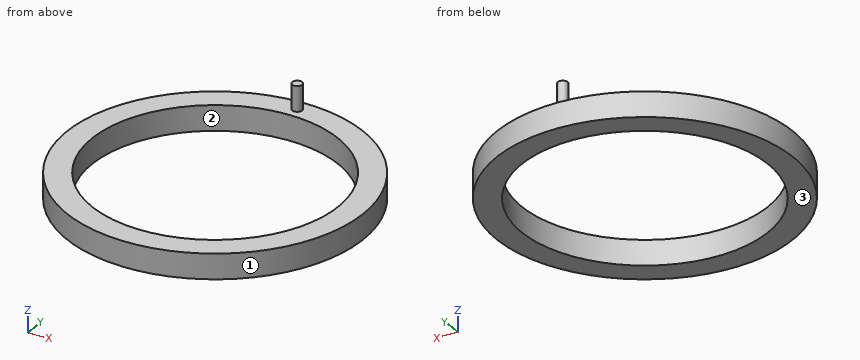
Autodesk Fusion 360 part; units mm, degrees
sketch "Sketch1" plane through (0, 0, 0) normal (0, 0, 1) x (1, 0, 0)
  circle A0 centre (0, 0) radius 29.5
  dimension "d1" = 59
sketch "Sketch2" plane through (0, 0, 0) normal (0, 0, 1) x (1, 0, 0)
  circle A0 centre (0, 0) radius 22.5
  dimension "d2" = 45
extrude "Extrude1" add sketch "Sketch1" sketch "Sketch2" along normal blind 5 of sketch 2
sketch "Sketch3" plane through (0, 0, 5) normal (0, 0, 1) x (-1, 0, 0)
  circle A0 centre (0, 0) radius 29.5
  circle A1 centre (0, 0) radius 24.5
  dimension "d5" = 49
extrude "Extrude2" cut sketch "Sketch3" against normal blind 115 contours A1
sketch "Sketch4" plane through (0, 0, 0) normal (0, 0, 1) x (1, 0, 0)
sketch "Sketch5" plane through (0, 0, 5) normal (0, 0, 1) x (-1, 0, 0)
  circle A0 centre (0, 0) radius 24.5
  circle A1 centre (0, 0) radius 29.5
  circle A2 centre (0, -27) radius 1
extrude "Extrude3" add sketch "Sketch5" along normal blind 5 contours A2
sketch "Sketch6" plane through (0, 0, 0) normal (0, 0, 1) x (1, 0, 0)
Here's how the part is built. I have some questions about the finished solid (model axes, mm). Face numbers are marked on the shaded views. Round coordinates to 2 decimals unless told otherwise and drop trailing zeros. Write each loop counter-clockwise with the first axis right and the second up, starting at its lowest first coordinate (ties: lowest second). Pieces come first, ordered by that corner, then holes.
Q1. If we section it at D-D on y = 27: Write out the boundary of the cut face in (x, z).
Q2. Please list where these lines run through material, in increasing order: probe 1 along Y at (x, z) = (0, 3.15); probe 2 along Z at (x, y) = (10.5, 23.5); probe 3 along Y at (x, z) = (18.5, 1).
Q3. If we section it at C-C on z = 3.25: Write out the boundary of the cut face in (x, y), plus the area to 3 significant figures.
Q4. If we section it at B-B on y = 0: Write out the boundary of the cut face in (x, z).
Q5. If we mould it in two halves opening along X, with no side actions, what happens to the marked faces 1, 2 and 3? For each: +X half, -X half, draft (parallel to the pull), parting line (faces both ways), or undercut.
Q6. Will these pins go through, and if not, where does the flat tip stop? P1, Ø2, axis at x = 20, z = 2, coming from the +Y side; P2, Ø5, axis at y = -16.5, z = 3, coming from the -X side; P3, Ø1, axis at x = -9, z = 2, coming from the -Y side.
Q7. If we section it at A-A on x = 0: Write out the boundary of the cut face in (y, z), plus the area to 3 significant figures.
Answer below:
1. outline: (-11.88, 0) - (11.88, 0) - (11.88, 5) - (1, 5) - (1, 10) - (-1, 10) - (-1, 5) - (-11.88, 5) - close
2. probe 1: y = -29.5 to -24.5, 24.5 to 29.5
2. probe 2: z = 0 to 5
2. probe 3: y = -22.98 to -16.06, 16.06 to 22.98
3. outline: circle Ø59 at (0, 0); hole circle Ø49 at (0, 0)
3. area: 848 mm2
4. outline: (-29.5, 0) - (-24.5, 0) - (-24.5, 5) - (-29.5, 5) - close; (24.5, 0) - (29.5, 0) - (29.5, 5) - (24.5, 5) - close
5. face 1: parting line
5. face 2: undercut
5. face 3: draft
6. P1: stops at y = 22.57
6. P2: stops at x = -25.97
6. P3: stops at y = -28.25
7. outline: (-29.5, 0) - (-24.5, 0) - (-24.5, 5) - (-29.5, 5) - close; (24.5, 0) - (29.5, 0) - (29.5, 5) - (28, 5) - (28, 10) - (26, 10) - (26, 5) - (24.5, 5) - close
7. area: 60.0 mm2
